Part model, mm, in its own coordinate system. Face numbers are marked on the shaded views. A direction names the side the tool comes from. Coordinates: 2 decimals unless noted, no trailing zeros. Order: outer loops, then holes, each group sorted by start corner. A loop starts at its lowest first (then second) coordinate and runs counter-clockwise, first axis right, second up.
1) Mould opens along Z. For the marked faces 4, 5 and 6 say: +Z half, -Z half, draft (parallel to the pull), parting line (faces both ways), or undercut.
2) Wall check: L1, parallel to Z at x = 20, y = -48.5; L2, parallel to Y at x = -7.5, z = 45; L3, parallel to X at y = -68, z = 61.5. Give the ranges that are in metal, low to high.
3) Pin check, flat tips, straight feed: pin 1 Ø1.5 at (y, z) = (20.5, 9.5) entering from -X; pin 2 Ø3 at (x, z) = (-6.5, 25.5) entering from +Y; pin 3 Ø8 at (y, z) = (20, 44) entering from -X. Stop position of each tip, or through.
4) Cut at C-C (x = 6). List the corners of the cut face in (y, z).
5) Cut at B-B (y = -25.5). List the corners of the cut face in (x, z), and give its area (3 significant figures).
6) Cut at D-D (z = 42). List the corners of the cut face in (x, y), and give its area (3 significant figures).
7) Tool access for the marked faces 1, 2 and 3: list every direction of +Z, -Z, +X, -X, +Y, -Y with a clear straight run to the whole face (end or side of a thin tool).
8) Cut at A-A (z = 18.5). List the corners of the cut face in (x, y).
```python
from build123d import *

# Parameters (mm, degrees)
F1_DEPTH = 70
F2_W     = 65.2701610255
F2_H     = 45.7058856264
F3_DEPTH = 127.5
F5_DEPTH = 41.3
F6_R     = 5
F7_R     = 8


with BuildPart() as f1:
    # F0 (on Top) → F1 (new body)
    with BuildSketch(Plane.XY):
        Polygon((-47.1203699708, 59.5582462847), (-58.6014762521, 59.5582462847), (-45.9271341588, 0), (-45.9271341588, -76.8745874723), (-37.5527814031, -77.7366533875), (-30.855467543, -12.6770474017), (11.2419202924, -12.6770474017), (21.7831026724, -78.1274641837), (30.8554805815, -77.7366533875), (27.5068189949, 0), (-33.725745976, 0), align=None)
    extrude(amount=F1_DEPTH)

    # F2 (on face) → F3 (cut)
    with BuildSketch(Plane(origin=(27.4558711207, 1.1827164786, 0), x_dir=(-0.0430370851, 0.9990734754, 0), z_dir=(0.9990734754, 0.0430370851, 0))):
        with Locations((-46.3574778998, 34.742649179)):
            Rectangle(F2_W, F2_H)
    extrude(amount=-F3_DEPTH, mode=Mode.SUBTRACT)

    # F4 (on face) → F5 (cut)
    with BuildSketch(Plane(origin=(-32.1020311258, -7.2197330046, 0), x_dir=(-0.2194189331, 0.9756307354, 0), z_dir=(0.9756307354, 0.2194189331, 0))):
        with BuildLine():
            Line((27.3875570842, 57.2867691517), (27.3875570842, 11.2720606849))
            ThreePointArc((27.3875570842, 11.2720606849), (53.1906745676, 34.2794149183), (27.3875570842, 57.2867691517))
        make_face()
    extrude(amount=-F5_DEPTH, mode=Mode.SUBTRACT)

    # F6
    f6_edges = [f1.edges().sort_by_distance(p)[0] for p in [
        (-3.109463, 0, 0),
        (-3.109463, 0, 70),
    ]]
    fillet(f6_edges, radius=F6_R)

    # F7
    f7_edges = [f1.edges().sort_by_distance(p)[0] for p in [
        (-47.12037, 59.558246, 35),
    ]]
    fillet(f7_edges, radius=F7_R)


solid = f1.part
```
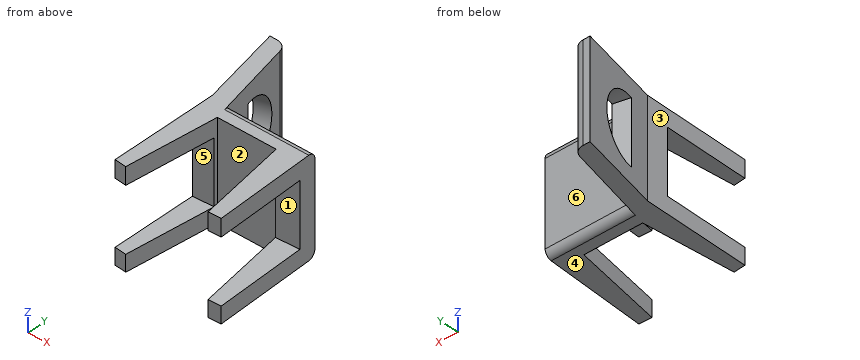
Geometry check:
1. face 4: -Z half
1. face 5: undercut
1. face 6: draft
2. L1: z = 0 to 11.89, 57.6 to 70
2. L2: y = -12.68 to 0
2. L3: x = -45.93 to -36.55, 20.15 to 30.44
3. pin 1: stops at x = -50.45
3. pin 2: stops at y = 0
3. pin 3: stops at x = -49.53
4. outline: (-12.68, 0) - (-5, 0) arc R5 ccw to (0, 5) - (0, 65) arc R5 ccw to (-5, 70) - (-12.68, 70) - close
5. outline: (-45.93, 0) - (-32.18, 0) - (-32.18, 11.89) - (-45.93, 11.89) - close; (-45.93, 57.6) - (-32.18, 57.6) - (-32.18, 70) - (-45.93, 70) - close; (13.31, 0) - (28.61, 0) - (28.61, 11.89) - (13.31, 11.89) - close; (13.31, 57.6) - (28.61, 57.6) - (28.61, 70) - (13.31, 70) - close
5. area: 706 mm2
6. outline: (-58.6, 59.56) - (-54.63, 40.88) - (-43.48, 43.38) - (-45.72, 53.31) arc R8 ccw to (-53.52, 59.56) - close; (-49.53, 16.93) - (-45.93, 0) - (-45.93, -15.71) - (-31.1, -15.07) - (-30.86, -12.68) - (11.24, -12.68) - (11.33, -13.25) - (28.05, -12.53) - (27.51, 0) - (-33.73, 0) - (-38.11, 19.5) - close
6. area: 1,390 mm2
7. face 1: +X, -Y
7. face 2: +Z, -Z, -Y
7. face 3: +Z, -Z, -X, -Y
8. outline: (-58.6, 59.56) - (-53.61, 36.1) - (-42.41, 38.62) - (-45.72, 53.31) arc R8 ccw to (-53.52, 59.56) - close; (-49.53, 16.93) - (-45.93, 0) - (-45.93, -15.71) - (-31.1, -15.07) - (-30.86, -12.68) - (11.24, -12.68) - (11.33, -13.25) - (28.05, -12.53) - (27.51, 0) - (-33.73, 0) - (-38.11, 19.5) - close
